Source: CAD feature listing. Evaluate the final solid. Frame: model axes, mm. Face numbers are marked on the shaded views. A direction names the side the tool comes from. Round coordinates to 2 decimals unless told otherwise and drop trailing zeros. Loops run counter-clockwise (first coordinate to the right, second up) from the corner with the lowest first, then second, coordinate; pieces in that order, holes last. Notation, with made-up numbers: (-6, 78) - (31, 78) arc R20 ccw to (31, 114) - close; hole circle Ø5 at (58.5, 17.25). An arc over 180 degrees is marked (long way). One line per question, with ' | ' between items. Start each with the question number.
1. Cut plane D-D (x = 11). Return loops of the section in (y, z), then the cut area to 3 significant figures.
2. Mould query, pull axis X, two halves, no side actions, for the marked faces 1, 2 and 3. Classes: pulls with the +X half, pulls with the -X half, needs draft (parallel to the pull), parting line crosses it, or undercut.
3. Access query for the marked faces 4 and 5. Directions: +Z, -Z, +X, -X, +Y, -Y. A direction counts if a zero-diameter tool reaches every point of the face in a straight line with its end or side. Return the directions, or none.
4. Cut plane B-B (x = 0). Return loops of the section in (y, z).
5. Cut plane A-A (z = 18). Return loops of the section in (x, y).
6. Ray query, line 1 (Y direction, x = -29, z = 9.25); line 2 (Y direction, x = 21.4, z = 3.25); line 3 (X direction, y = 7, z = 28). Return the intervals inside material, ascending.
7. Pin query (flat end, axial travel): pin 1 (3.5 mm diameter, centred on x = -21, y = -5.5, fed in from +Z); pin 2 (2.5 mm diameter, centred on x = 29, y = -26, fed in from +Z); pin 3 (11.5 mm diameter, centred on x = 0, z = 18, fed in from +Y); pin 4 (0.9 mm diameter, centred on x = -21, y = 6, fed in from +Z). Return the tip coordinate at first contact, or that it passes through.
8. Cut plane C-C (z = 6). State how many separate pieces and enclosed holes the cut face has, then the cut area to 3 significant figures.
```python
from build123d import *

# Parameters (mm, degrees)
SKETCH_W        = 66
SKETCH_H        = 60
PAD_DEPTH       = 30
FILLET_R        = 4
SKETCH001_R     = 1.35
POCKET_DEPTH    = 27
POCKET001_DEPTH = 20
SKETCH003_R     = 1.5
POCKET002_DEPTH = 9.5
SKETCH004_R     = 6.5
POCKET003_DEPTH = 60.001


with BuildPart() as part:
    # Sketch → Pad (new body)
    with BuildSketch(Plane.XY):
        Rectangle(SKETCH_W, SKETCH_H)
    extrude(amount=PAD_DEPTH)

    # Fillet
    fillet_edges = [part.edges().sort_by_distance(p)[0] for p in [
        (-33, -30, 15),
        (33, -30, 15),
        (33, 30, 15),
        (-33, 30, 15),
    ]]
    fillet(fillet_edges, radius=FILLET_R)

    # Sketch001 (on Face5 of Fillet) → Pocket (cut)
    with BuildSketch(Plane.XY.offset(30)):
        with Locations((-29, 26)):
            Circle(SKETCH001_R)
        with Locations((29, 26)):
            Circle(SKETCH001_R)
        with Locations((29, -26)):
            Circle(SKETCH001_R)
        with Locations((-29, -26)):
            Circle(SKETCH001_R)
    extrude(amount=-POCKET_DEPTH, mode=Mode.SUBTRACT)

    # Sketch002 (on Face5 of Pocket) → Pocket001 (cut)
    with BuildSketch(Plane.XY.offset(30)):
        with BuildLine():
            ThreePointArc((-30, 23.171573), (-26.87868, 23.87868), (-26.171573, 27))
            Line((26.171573, 27), (-26.171573, 27))
            ThreePointArc((26.171573, 27), (26.87868, 23.87868), (30, 23.171573))
            Line((30, -23.171573), (30, 23.171573))
            ThreePointArc((30, -23.171573), (26.87868, -23.87868), (26.171573, -27))
            Line((-26.171573, -27), (26.171573, -27))
            ThreePointArc((-26.171573, -27), (-26.87868, -23.87868), (-30, -23.171573))
            Line((-30, 23.171573), (-30, -23.171573))
        make_face()
    extrude(amount=-POCKET001_DEPTH, mode=Mode.SUBTRACT)

    # Sketch003 (on Face26 of Pocket001) → Pocket002 (cut)
    with BuildSketch(Plane.XY.offset(10)):
        with Locations((-21.4, 6.35)):
            Circle(SKETCH003_R)
        with Locations((21.4, 6.35)):
            Circle(SKETCH003_R)
        with Locations((21.4, -6.35)):
            Circle(SKETCH003_R)
        with Locations((-21.4, -6.35)):
            Circle(SKETCH003_R)
    extrude(amount=-POCKET002_DEPTH, mode=Mode.SUBTRACT)

    # Sketch004 (on Face6 of Pocket002) → Pocket003 (cut, through all)
    with BuildSketch(Plane.XZ.offset(30)):
        with Locations((0, 18)):
            Circle(SKETCH004_R)
    extrude(amount=-POCKET003_DEPTH, mode=Mode.SUBTRACT)


solid = part.part
```
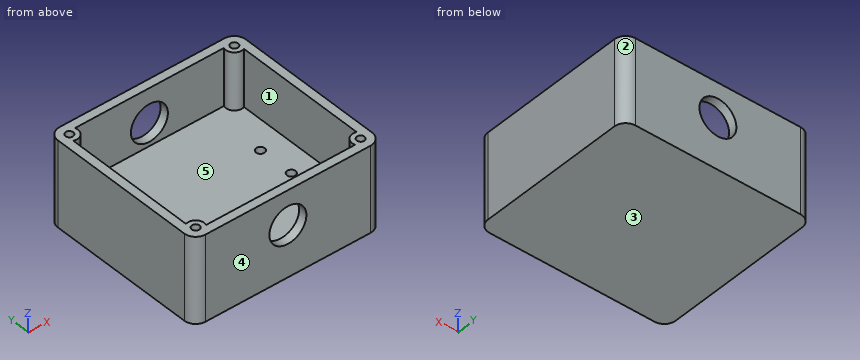
Answers follow:
1) outline: (-30, 0) - (30, 0) - (30, 30) - (27, 30) - (27, 10) - (-27, 10) - (-27, 30) - (-30, 30) - close | area: 720 mm2
2) face 1: undercut | face 2: pulls with the +X half | face 3: needs draft
3) face 4: +Z, -Z, +X, -X, -Y | face 5: +Z
4) outline: (-30, 0) - (30, 0) - (30, 11.5) - (27, 11.5) - (27, 10) - (-27, 10) - (-27, 11.5) - (-30, 11.5) - close; (-30, 24.5) - (-27, 24.5) - (-27, 30) - (-30, 30) - close; (27, 24.5) - (30, 24.5) - (30, 30) - (27, 30) - close
5) outline: (-33, -26) arc R4 ccw to (-29, -30) - (-6.5, -30) - (-6.5, -27) - (-26.17, -27) arc R3 ccw to (-30, -23.17) - (-30, 23.17) arc R3 ccw to (-26.17, 27) - (-6.5, 27) - (-6.5, 30) - (-29, 30) arc R4 ccw to (-33, 26) - close; (6.5, -30) - (29, -30) arc R4 ccw to (33, -26) - (33, 26) arc R4 ccw to (29, 30) - (6.5, 30) - (6.5, 27) - (26.17, 27) arc R3 ccw to (30, 23.17) - (30, -23.17) arc R3 ccw to (26.17, -27) - (6.5, -27) - close; hole circle Ø2.7 at (-29, -26); hole circle Ø2.7 at (-29, 26); hole circle Ø2.7 at (29, -26); hole circle Ø2.7 at (29, 26)
6) line 1: y = -30 to -27.35, -24.65 to 24.65, 27.35 to 30 | line 2: y = -30 to -7.85, -4.85 to 4.85, 7.85 to 30 | line 3: x = -33 to -30, 30 to 33
7) pin 1: stops at z = 10 | pin 2: stops at z = 3 | pin 3: passes through | pin 4: stops at z = 0.5
8) separate pieces: 1 | enclosed holes: 8 | area: 3,900 mm2
